```python
from build123d import *

# Parameters (mm, degrees)
F0_W          = 45
F0_H          = 45
F1_DEPTH      = 2795
F3_W          = 45
F3_H          = 60
F3_W_2        = 90
F3_W_3        = 15
F4_DEPTH      = 5
F6_DEPTH      = 45
F8_W          = 2.7798460424
F8_H          = 5.7082939148
F9_DEPTH      = 156.8
F9_DEPTH_BACK = 105
F14_DEPTH     = 5
F15_DEPTH     = 30


with BuildPart() as f1:
    # F0 (on Top) → F1 (new body)
    with BuildSketch(Plane.XY):
        Rectangle(F0_W, F0_H)
    extrude(amount=F1_DEPTH)


with BuildPart() as f4:
    # F3 (on face) → F4 (new body)
    with BuildSketch(Plane(origin=(0, -524.3318959349, 2697.453760933), x_dir=(1, 0, 0), z_dir=(0, -0.1908089954, 0.9816271834))):
        with Locations((-15, 541.2245304499)):
            Rectangle(F3_W, F3_H)
        with Locations((-82.5, 541.2245304499)):
            Rectangle(F3_W_2, F3_H)
        with Locations((15, 541.2245304499)):
            Rectangle(F3_W_3, F3_H)
        Polygon((-37.5, 661.2245304499), (-37.5, 571.2245304499), (7.5, 571.2245304499), (22.5, 571.2245304499), (22.5, 661.2245304499), align=None)
    extrude(amount=F4_DEPTH)


with BuildPart() as f6:
    # F5 (on face) → F6 (new body)
    with BuildSketch(Plane.YZ.offset(22.5)):
        Polygon((-22.5, 2795), (22.5, 2795), (22.5, 2803.7471139112), align=None)
    extrude(amount=-F6_DEPTH)


with BuildPart() as f1_1:
    add(f1.part)

    # F7: union F6, F4
    add(f6.part)
    add(f4.part)

    # F8 (on face) → F9 (cut, two sides)
    with BuildSketch(Plane(origin=(-22.5, 0, 0), x_dir=(0, -1, 0), z_dir=(-1, 0, 0))) as f9_sk:
        with Locations((23.8899230212, 2797.8541469574)):
            Rectangle(F8_W, F8_H)
    extrude(amount=-F9_DEPTH, mode=Mode.SUBTRACT)
    extrude(f9_sk.sketch, amount=F9_DEPTH_BACK, mode=Mode.SUBTRACT)

    # F13 (on face) → F14 (cut, through all)
    with BuildSketch(Plane(origin=(0, -525.2859409117, 2702.3618968503), x_dir=(1, 0, 0), z_dir=(0, -0.1908089954, 0.9816271834))):
        with BuildLine():
            ThreePointArc((-56.5, 556.2245304499), (-66.7426406871, 560.467171137), (-62.5, 550.2245304499))
            ThreePointArc((-62.5, 550.2245304499), (-58.2573593129, 551.9818897628), (-56.5, 556.2245304499))
        make_face()
        with BuildLine():
            ThreePointArc((-96.5, 556.2245304499), (-102.5, 562.2245304499), (-108.5, 556.2245304499))
            ThreePointArc((-108.5, 556.2245304499), (-102.5, 550.2245304499), (-96.5, 556.2245304499))
        make_face()
        with BuildLine():
            ThreePointArc((-16.5, 596.2245304499), (-26.7426406871, 600.467171137), (-22.5, 590.2245304499))
            ThreePointArc((-22.5, 590.2245304499), (-18.2573593129, 591.9818897628), (-16.5, 596.2245304499))
        make_face()
        with BuildLine():
            ThreePointArc((-16.5, 636.2245304499), (-18.2573593129, 640.467171137), (-22.5, 642.2245304499))
            ThreePointArc((-22.5, 642.2245304499), (-26.7426406871, 631.9818897628), (-16.5, 636.2245304499))
        make_face()
    extrude(amount=-F14_DEPTH, mode=Mode.SUBTRACT)

    # F12 (on offset) → F15 (join)
    with BuildSketch(Plane.XY.offset(2545)):
        with BuildLine():
            Line((0, 27.5), (5, 27.5))
            ThreePointArc((5, 27.5), (0, 32.5), (-5, 27.5))
            Line((-5, 27.5), (0, 27.5))
        make_face()
        with BuildLine():
            Line((5, 22.5), (5, 27.5))
            ThreePointArc((5, 27.5), (3.5355339059, 23.9644660941), (0, 22.5))
            Line((0, 22.5), (5, 22.5))
        make_face()
        with BuildLine():
            ThreePointArc((0, 22.5), (3.5355339059, 23.9644660941), (5, 27.5))
            Line((5, 27.5), (0, 27.5))
            Line((0, 27.5), (0, 22.5))
        make_face()
        with BuildLine():
            Line((0, 27.5), (-5, 27.5))
            ThreePointArc((-5, 27.5), (-3.5355339059, 23.9644660941), (0, 22.5))
            Line((0, 22.5), (0, 27.5))
        make_face()
        with BuildLine():
            ThreePointArc((0, 22.5), (-3.5355339059, 23.9644660941), (-5, 27.5))
            Line((-5, 27.5), (-5, 22.5))
            Line((-5, 22.5), (0, 22.5))
        make_face()
    extrude(amount=F15_DEPTH)

    # F17: sweep along a path in F11
    with BuildLine(Plane.YZ) as f17_path:
        ThreePointArc((57.5, 2575), (42.5, 2590), (27.5, 2575))
    # F16 (on face) → F17 (sweep)
    with BuildSketch(Plane.XY.offset(2575)):
        with BuildLine():
            ThreePointArc((0, 22.5), (3.5355339059, 23.9644660941), (5, 27.5))
            ThreePointArc((5, 27.5), (0, 32.5), (-5, 27.5))
            ThreePointArc((-5, 27.5), (-3.5355339059, 23.9644660941), (0, 22.5))
        make_face()
    sweep(path=f17_path.line)


solid = f1_1.part
```
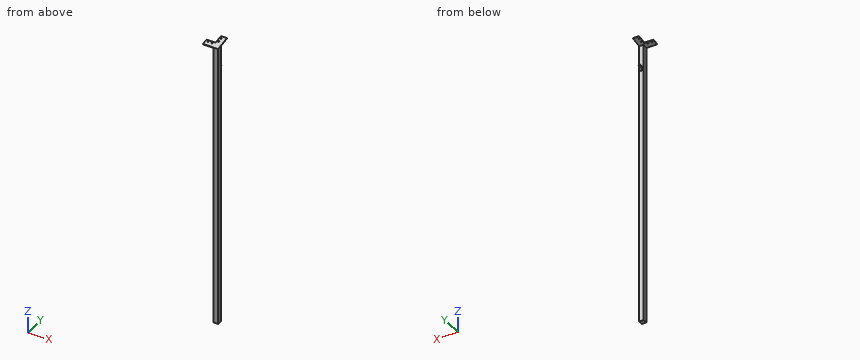
Input: part model. Units: mm. Frame: model coordinates. Give positions to 0.01 mm unless a question says otherwise; leave off trailing zeros. Order: outer loops, then holes, each group sorted by start corner. A loop starts at its lowest first (then second) coordinate and runs counter-clockwise, first axis right, second up. Notation, with made-up numbers: (22.5, 59.5) - (64.5, 59.5) arc R25 cw to (64.5, 84.5) - close; hole circle Ø8 at (44.25, 29.5). An arc over 180 degrees is marked (long way). Put each result on its own line as item: value.
Item 1: Contact query for flat-ended pins moving along their axis: pin 1 (1.5 mm diameter, centred on y = 25.5, z = 2560, fed in from +X); pin 2 (17.5 mm diameter, centred on y = 90.5, z = 2822, fed in from -X); pin 3 (4 mm diameter, centred on x = 1.5, y = 25, fed in from +Z). Output: stop coordinate, or through.
Found:
pin 1: stops at x = 5
pin 2: stops at x = -37.5
pin 3: stops at z = 2809.72
Item 2: Section query A-A, the plane z = 2178.5. Return loops of the section in (x, y), then the cut area to 4 significant figures.
Found:
outline: (-22.5, -22.5) - (22.5, -22.5) - (22.5, 22.5) - (-22.5, 22.5) - close
area: 2,025 mm^2
Item 3: Ray query, L1, parallel to Y at x = -6, z = 2380; L2, parallel to Z at x = -32, y = 20.5. Return the intervals inside material, ascending. Write a range as from..to.
Found:
L1: y = -22.5..22.5
L2: z = 2803.36..2808.45
